Check sheet for the drawn part. Datum: minimum x, y, z corner. Units: mm. A direction names the side the tool comes from. Give positions to 0.01 mm unless a question says otherwise; leave off trailing zeros. Order: outer loops, then holes, each group sorted by start corner. A loop starts at its lowest first (then second) coordinate and runs counter-clockwise, first axis right, second up. Notation, with made-up numbers: (83, -18) -> (90, -18) arc R5 ccw to (90, -9) -> close; hole circle Ø5 at (43.5, 21.5). An arc over 180 degrees is marked (long way). One line per question, with ' | ' between items. Start each with the question number.
Q1. Section check C-C on z = 9. Record the cut outline in (x, y), plus the area to 3 significant figures.
Q2. Access from +Z, -Z, +X, -X, +Y, -Y to the whole of each face (thin tool, end or side, straight path). Record for the marked faces 1 and 2.
Q3. Section check D-D on y = 18. Record the cut outline in (x, z).
Q4. Go/stop test with flat-tipped pins: pin 1 (12 mm diameter, centred on x = 34.5, z = 12.5, fed in from +Y); pin 2 (6 mm diameter, centred on x = 33, z = 24.5, fed in from +Y); pin 3 (1 mm diameter, centred on y = 47, z = 8.5, fed in from +X). Record where each tip stops, or that it passes through.
Q5. Mould release check, pull along X, two halves, no side actions. Record for the marked faces 3, 4 and 5: released by +X, released by -X, zero draft, split by the parting line, or undercut.
Q6. Section check A-A on y = 27. Record the cut outline in (x, z), plus the area to 3 significant figures.
Q7. Material ranges on probe 1 along Y at (x, z) = (27, 20.75); probe 2 along Y at (x, z) = (27, 7); probe 3 along X at (y, z) = (27.5, 25.5), recorded low to high. Write a range as [from, to].
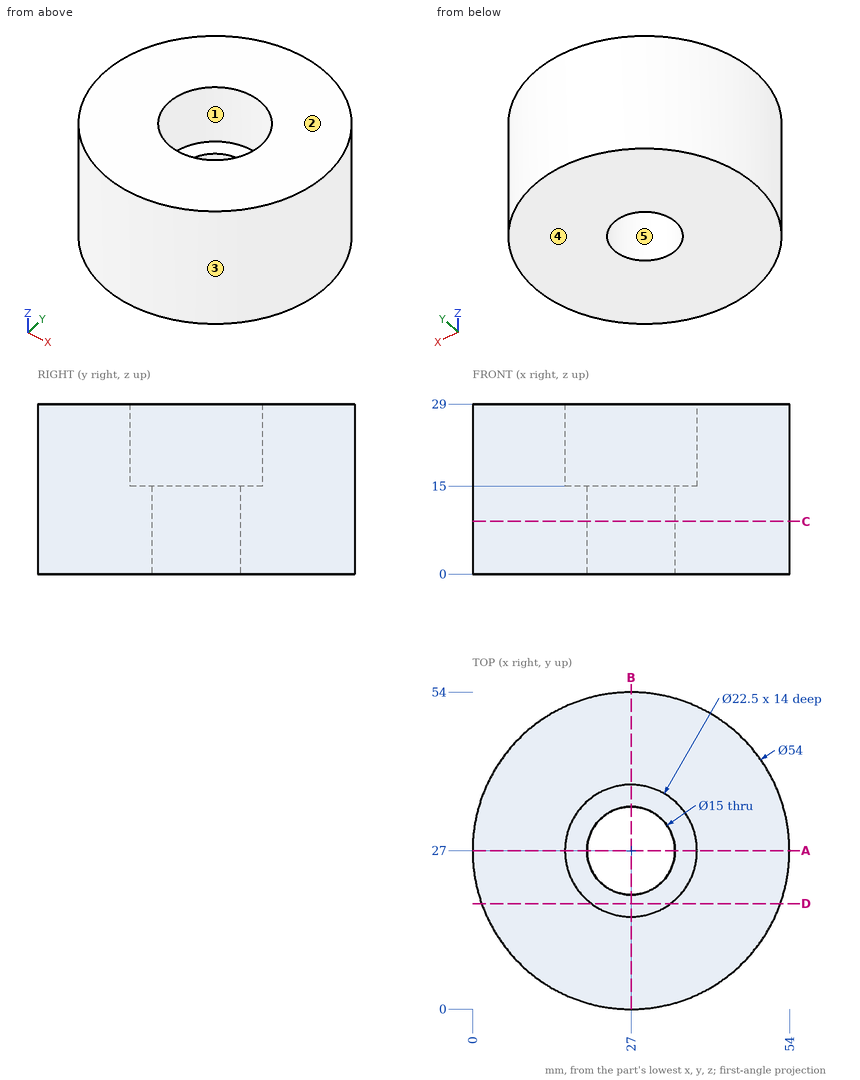
Filled in:
1) outline: circle Ø54 at (27, 27); hole circle Ø15 at (27, 27) | area: 2,110 mm²
2) face 1: +Z | face 2: +Z, +X, -X, +Y, -Y
3) outline: (1.54, 0) -> (52.46, 0) -> (52.46, 29) -> (33.75, 29) -> (33.75, 15) -> (20.25, 15) -> (20.25, 29) -> (1.54, 29) -> close
4) pin 1: y = 53.96 | pin 2: y = 53.83 | pin 3: x = 45.67
5) face 3: split by the parting line | face 4: zero draft | face 5: undercut
6) outline: (0, 0) -> (19.5, 0) -> (19.5, 15) -> (15.75, 15) -> (15.75, 29) -> (0, 29) -> close; (34.5, 0) -> (54, 0) -> (54, 29) -> (38.25, 29) -> (38.25, 15) -> (34.5, 15) -> close | area: 1,030 mm²
7) probe 1: [0, 15.75], [38.25, 54] | probe 2: [0, 19.5], [34.5, 54] | probe 3: [0, 15.76], [38.24, 54]
